Design review of the part built by this model. Coordinates are the model's own, in mm. A direction names the side the tool comes from. Coordinates: 2 decimals unless noted, no trailing zeros. Order: outer loops, then holes, each group sorted by start corner. A loop starts at its lowest first (then second) coordinate and runs counter-clockwise, first axis right, second up. Notation, with made-up numbers: (1.25, -30.75) -> (14.25, -30.75) arc R21 ccw to (14.25, -16.75) -> close; hole circle Ø2 at (3.25, 17). An arc over 180 degrees is marked (long way). Use a Markdown table: item, result. Add a question column.
Q1. Wall thickness on probe 1 along Y at (x, z) = (-29, -1.4); probe 2 along Y at (x, z) = (4.5, -1.4); probe 3 along X at (y, z) = (9, -1.4): over which ranges is each line inside the solid? List them lowest first.
Q2. Add section D-D (y = -4). State the section outline as (x, z) points, then the cut area to 3 significant figures.
Q3. Add section B-B (z = -0.45). Count the separate pieces of the cut face and the enclosed holes in it, then the cut area to 3 significant figures.
Q4. Add section C-C (x = 14.5). State the section outline as (y, z) points.
Q5. Machinability: for faces 4 (the face through (6, -5.75, -1)), 5 (the face through (31.1, 11.14, -0.76)), which of the approach directions +Z, -Z, +X, -X, +Y, -Y give a long, thin tool a straight path to every point of the face, cutting with its end or side? Answer none if there is none.
Q6. The part is to be moulded in two halves that separate along X. For faces 1 (the face through (-32, -2, -1)), 2 (the face through (0, 12, -1)), 3 (the face through (1.5, -4, -1)), say which applies: pulls with the +X half, pulls with the -X half, needs draft (parallel to the pull), parting line crosses it, or undercut.
Q7. Insertion check: pin 1 (6 mm diameter, centred on x = -21, y = 1, fed in from -Z); pin 2 (3.5 mm diameter, centred on x = -29, y = 9, fed in from +Z). Each pin has a flat end and moves straight along its axis. Give the tip position at first contact, or say it passes through.
Q8. Add section A-A (x = 22). State the section outline as (y, z) points, then the cut area to 3 significant figures.
from build123d import *

# Parameters (mm, degrees)
SKETCH1_W                                      = 64
SKETCH1_H                                      = 24
BOSS_EXTRUDE1_DEPTH                            = 1.5
CSK_FOR_M2_5_FLAT_HEAD_MACHINE_SCREW1_AT_COUNT = 2
CSK_FOR_M2_5_FLAT_HEAD_MACHINE_SCREW1_AT_PITCH = 58
CSK_FOR_M2_5_FLAT_HEAD_MACHINE_SCREW_2_COUNT   = 2
CSK_FOR_M2_5_FLAT_HEAD_MACHINE_SCREW_2_PITCH   = 18
CSK_FOR_M2_5_FLAT_HEAD_MACHINE_SCREW_3_COUNT   = 2
CSK_FOR_M2_5_FLAT_HEAD_MACHINE_SCREW_3_PITCH   = 60.728905803
FILLET1_R                                      = 3
SKETCH4_R                                      = 3.3
CUT_EXTRUDE1_DEPTH                             = 35.208916966
SKETCH5_R                                      = 1.6
CUT_EXTRUDE2_DEPTH                             = 35.208916966
SKETCH6_R                                      = 1.9
CUT_EXTRUDE3_DEPTH                             = 35.208916966
SKETCH7_W                                      = 9
SKETCH7_H                                      = 4
CUT_EXTRUDE4_DEPTH                             = 35.208916966


with BuildPart() as part:
    # Sketch1 → Boss-Extrude1 (new body)
    with BuildSketch(Plane.XY):
        Rectangle(SKETCH1_W, SKETCH1_H)
    extrude(amount=-BOSS_EXTRUDE1_DEPTH)

    # Sketch2 → CSK for M2.5 Flat Head Machine Screw1 (revolve, cut)
    with BuildSketch(Plane(origin=(-29, 9, 0), x_dir=(0, -1, 0), z_dir=(1, 0, 0))):
        Polygon((0, 0), (0, 1.5), (1.45, 1.5), (1.45, 1.3), (2.75, 0), align=None)
    csk_for_m2_5_flat_head_machine_screw1 = revolve(axis=Axis((-29, 9, 6.35), (0, 0, -1)), mode=Mode.SUBTRACT)

    # CSK for M2.5 Flat Head Machine Screw1 at: CSK for M2.5 Flat Head Machine Screw1 ×2
    with Locations(*[(i * CSK_FOR_M2_5_FLAT_HEAD_MACHINE_SCREW1_AT_PITCH, 0, 0) for i in range(1, CSK_FOR_M2_5_FLAT_HEAD_MACHINE_SCREW1_AT_COUNT)]):
        add(csk_for_m2_5_flat_head_machine_screw1, mode=Mode.SUBTRACT)

    # CSK for M2.5 Flat Head Machine Screw 2: CSK for M2.5 Flat Head Machine Screw1 ×2
    with Locations(*[(0, -i * CSK_FOR_M2_5_FLAT_HEAD_MACHINE_SCREW_2_PITCH, 0) for i in range(1, CSK_FOR_M2_5_FLAT_HEAD_MACHINE_SCREW_2_COUNT)]):
        add(csk_for_m2_5_flat_head_machine_screw1, mode=Mode.SUBTRACT)

    # CSK for M2.5 Flat Head Machine Screw 3: CSK for M2.5 Flat Head Machine Screw1 ×2
    with Locations(*[Vector(0.9550641368112371, -0.2963992148724529, 0) * (i * CSK_FOR_M2_5_FLAT_HEAD_MACHINE_SCREW_3_PITCH) for i in range(1, CSK_FOR_M2_5_FLAT_HEAD_MACHINE_SCREW_3_COUNT)]):
        add(csk_for_m2_5_flat_head_machine_screw1, mode=Mode.SUBTRACT)

    # Fillet1
    fillet1_edges = [part.edges().sort_by_distance(p)[0] for p in [
        (-32, 12, -0.75),
        (32, 12, -0.75),
    ]]
    fillet(fillet1_edges, radius=FILLET1_R)

    # Sketch4 → Cut-Extrude1 (cut, through all)
    with BuildSketch(Plane.XY):
        with Locations((-21, 1)):
            Circle(SKETCH4_R)
    extrude(amount=-CUT_EXTRUDE1_DEPTH, mode=Mode.SUBTRACT)

    # Sketch5 → Cut-Extrude2 (cut, through all)
    with BuildSketch(Plane.XY):
        with Locations((14.5, -3)):
            Circle(SKETCH5_R)
    extrude(amount=-CUT_EXTRUDE2_DEPTH, mode=Mode.SUBTRACT)

    # Sketch6 → Cut-Extrude3 (cut, through all)
    with BuildSketch(Plane.XY):
        with Locations((22, -1)):
            Circle(SKETCH6_R)
    extrude(amount=-CUT_EXTRUDE3_DEPTH, mode=Mode.SUBTRACT)

    # Sketch7 → Cut-Extrude4 (cut, through all)
    with BuildSketch(Plane.XY):
        with Locations((6, -3.75)):
            Rectangle(SKETCH7_W, SKETCH7_H)
    extrude(amount=-CUT_EXTRUDE4_DEPTH, mode=Mode.SUBTRACT)


solid = part.part
Established:
| question | item | result |
|---|---|---|
| 1 | probe 1 | -12 to -10.45, -7.55 to 7.55, 10.45 to 12 |
| 1 | probe 2 | -12 to -5.75, -1.75 to 12 |
| 1 | probe 3 | -32 to -30.45, -27.55 to 27.55, 30.45 to 32 |
| 2 | outline | (-32, -1.5) -> (1.5, -1.5) -> (1.5, 0) -> (-32, 0) -> close; (10.5, -1.5) -> (13.25, -1.5) -> (13.25, 0) -> (10.5, 0) -> close; (15.75, -1.5) -> (32, -1.5) -> (32, 0) -> (15.75, 0) -> close |
| 2 | area | 78.8 mm^2 |
| 3 | separate pieces | 1 |
| 3 | enclosed holes | 8 |
| 3 | area | 1,380 mm^2 |
| 4 | outline | (-12, -1.5) -> (-4.6, -1.5) -> (-4.6, 0) -> (-12, 0) -> close; (-1.4, -1.5) -> (12, -1.5) -> (12, 0) -> (-1.4, 0) -> close |
| 5 | face 4 | +Z, -Z |
| 5 | face 5 | +Z, -Z, +X, +Y |
| 6 | face 1 | pulls with the -X half |
| 6 | face 2 | needs draft |
| 6 | face 3 | undercut |
| 7 | pin 1 | through |
| 7 | pin 2 | z = -1 |
| 8 | outline | (-12, -1.5) -> (-2.9, -1.5) -> (-2.9, 0) -> (-12, 0) -> close; (0.9, -1.5) -> (12, -1.5) -> (12, 0) -> (0.9, 0) -> close |
| 8 | area | 30.3 mm^2 |
